```python
from build123d import *

# Parameters (mm, degrees)
SKETCH3_W           = 38.1
SKETCH3_H           = 38.1
BOSS_EXTRUDE2_DEPTH = 3.81
FILLET1_R           = 3.175
CUT_EXTRUDE1_REACH  = 65.074
SKETCH4_R           = 1.627
FILLET2_R           = 1.27
CUT_EXTRUDE2_REACH  = 64.728
SKETCH5_R           = 1.905
SKETCH7_W           = 6.35
SKETCH7_H           = 6.35
CUT_EXTRUDE4_DEPTH  = 5.08


with BuildPart() as part:
    # Sketch3 → Boss-Extrude2 (new, symmetric)
    with BuildSketch(Plane.XY):
        Polygon((34.29, -3.175), (34.29, 3.175), (26.67, 3.175), (26.67, 41.275), (34.29, 41.275), (34.29, 47.625), (13.97, 47.625), (13.97, 52.3875), (4.445, 52.3875), (4.445, 47.625), (-4.445, 47.625), (-4.445, 52.3875), (-13.97, 52.3875), (-13.97, 47.625), (-34.29, 47.625), (-34.29, 41.275), (-26.67, 41.275), (-26.67, 3.175), (-34.29, 3.175), (-34.29, -3.175), (-19.05, -3.175), (-19.05, 0), (19.05, 0), (19.05, -3.175), align=None)
        with Locations((0, 22.225)):
            Rectangle(SKETCH3_W, SKETCH3_H, mode=Mode.SUBTRACT)
    extrude(amount=BOSS_EXTRUDE2_DEPTH, both=True)

    # Fillet1
    fillet1_edges = [part.edges().sort_by_distance(p)[0] for p in [
        (34.29, 3.175, 0),
        (34.29, 41.275, 0),
        (34.29, 47.625, 0),
        (-34.29, 3.175, 0),
        (-34.29, 41.275, 0),
        (34.29, -3.175, 0),
        (-34.29, -3.175, 0),
        (-34.29, 47.625, 0),
    ]]
    fillet(fillet1_edges, radius=FILLET1_R - 0.0001)  # a hair under: the kernel refuses the full size

    # Sketch4 → Cut-Extrude1 (cut, up to next)
    with BuildSketch(Plane.XY.offset(3.81), mode=Mode.PRIVATE) as cut_extrude1_sk1:
        with Locations((-31.115, 44.45)):
            Circle(SKETCH4_R)
    cut_extrude1_tool1 = extrude(cut_extrude1_sk1.sketch, amount=-CUT_EXTRUDE1_REACH, mode=Mode.PRIVATE) & part.part
    # Sketch4 → Cut-Extrude1 (cut, up to next)
    with BuildSketch(Plane.XY.offset(3.81), mode=Mode.PRIVATE) as cut_extrude1_sk2:
        with Locations((-31.115, 0)):
            Circle(SKETCH4_R)
    cut_extrude1_tool2 = extrude(cut_extrude1_sk2.sketch, amount=-CUT_EXTRUDE1_REACH, mode=Mode.PRIVATE) & part.part
    cut_extrude1_1 = cut_extrude1_tool1.solids().sort_by_distance((-31.115, 44.45, 3.81))[0]
    add(cut_extrude1_1, mode=Mode.SUBTRACT)
    cut_extrude1_2 = cut_extrude1_tool2.solids().sort_by_distance((-31.115, 0, 3.81))[0]
    add(cut_extrude1_2, mode=Mode.SUBTRACT)
    cut_extrude1 = cut_extrude1_1 + cut_extrude1_2  # Cut-Extrude1 as one shape, for the pattern or mirror that repeats it

    # Mirror1: Cut-Extrude1 across plane
    add(cut_extrude1.mirror(Plane(origin=(0, 0, 0), x_dir=(0, 0, 1), z_dir=(1, 0, 0))), mode=Mode.SUBTRACT)

    # Fillet2
    fillet2_edges = [part.edges().sort_by_distance(p)[0] for p in [
        (-26.67, 22.225, -3.81),
        (26.67, 22.225, -3.81),
        (-13.97, 47.625, 0),
        (-13.97, 52.3875, 0),
        (-4.445, 52.3875, 0),
        (-4.445, 47.625, 0),
        (4.445, 52.3875, 0),
        (13.97, 52.3875, 0),
        (26.67, 22.225, 3.81),
        (13.97, 47.625, 0),
        (-19.05, 22.225, -3.81),
        (0, 3.175, -3.81),
        (-19.05, 3.175, 0),
        (19.05, 22.225, -3.81),
        (19.05, 3.175, 0),
        (-19.05, 22.225, 3.81),
        (0, 3.175, 3.81),
        (19.05, 22.225, 3.81),
        (-26.67, 22.225, 3.81),
    ]]
    fillet(fillet2_edges, radius=FILLET2_R)

    # Sketch5 → Cut-Extrude2 (cut, up to next)
    with BuildSketch(Plane.XZ, mode=Mode.PRIVATE) as cut_extrude2_sk1:
        with Locations((-15.24, 0)):
            Circle(SKETCH5_R)
    cut_extrude2_tool1 = extrude(cut_extrude2_sk1.sketch, amount=-CUT_EXTRUDE2_REACH, mode=Mode.PRIVATE) & part.part
    # Sketch5 → Cut-Extrude2 (cut, up to next)
    with BuildSketch(Plane.XZ, mode=Mode.PRIVATE) as cut_extrude2_sk2:
        with Locations(Location((15.24, 0, 0), (0, 0, 180))):
            Circle(SKETCH5_R)
    cut_extrude2_tool2 = extrude(cut_extrude2_sk2.sketch, amount=-CUT_EXTRUDE2_REACH, mode=Mode.PRIVATE) & part.part
    add(cut_extrude2_tool1.solids().sort_by_distance((-15.24, 0, 0))[0], mode=Mode.SUBTRACT)
    add(cut_extrude2_tool2.solids().sort_by_distance((15.24, 0, 0))[0], mode=Mode.SUBTRACT)

    # Sketch7 → Cut-Extrude4 (cut)
    with BuildSketch(Plane.XY.offset(3.81)):
        with Locations((-9.2075, 47.625)):
            Rectangle(SKETCH7_W, SKETCH7_H)
    cut_extrude4 = extrude(amount=-CUT_EXTRUDE4_DEPTH, mode=Mode.SUBTRACT)

    # Mirror2: Cut-Extrude4 across plane
    add(cut_extrude4.mirror(Plane(origin=(0, 0, 0), x_dir=(0, 0, 1), z_dir=(1, 0, 0))), mode=Mode.SUBTRACT)


solid = part.part
```
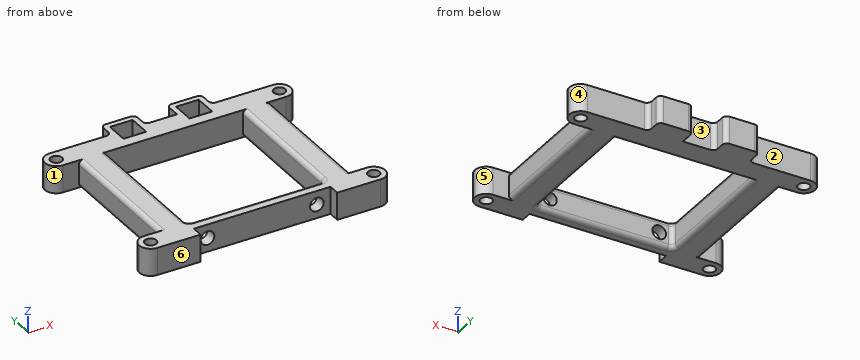
Check sheet for the modelled part. Datum: model origin and axes. Units: mm. Face numbers are marked on the shaded views. A direction names the side the tool comes from. Coordinates: 2 decimals unless noted, no trailing zeros. Write each loop counter-clockwise with the first axis right and the second up, starting at its lowest first coordinate (ties: lowest second). Pieces come first, ordered by that corner, then holes. Notation, with made-up numbers: (68.5, -21.75) -> (81.5, -21.75) arc R10 cw to (81.5, -10.75) -> close; hole circle Ø11 at (76, 16.5). An arc over 180 degrees is marked (long way). Use a Markdown table: item, result.
1. Sectioned sample at A-A (y = 22). Enter the section's corners in (x, z).
Reported:
| item | result |
|---|---|
| outline | (-26.67, -2.54) arc R1.27 ccw to (-25.4, -3.81) -> (-20.32, -3.81) arc R1.27 ccw to (-19.05, -2.54) -> (-19.05, 2.54) arc R1.27 ccw to (-20.32, 3.81) -> (-25.4, 3.81) arc R1.27 ccw to (-26.67, 2.54) -> close; (19.05, -2.54) arc R1.27 ccw to (20.32, -3.81) -> (25.4, -3.81) arc R1.27 ccw to (26.67, -2.54) -> (26.67, 2.54) arc R1.27 ccw to (25.4, 3.81) -> (20.32, 3.81) arc R1.27 ccw to (19.05, 2.54) -> close |
2. Release check for a two-part mould opening along Y. For the marked faces 4, 5 and 6 record: pulls with the +Y half, pulls with the -Y half, needs draft (parallel to the pull), parting line crosses it, or undercut.
Reported:
| item | result |
|---|---|
| face 4 | pulls with the +Y half |
| face 5 | undercut |
| face 6 | pulls with the -Y half |
3. Scan lines: line 1 along Y through (x, z) = (-31, -3) (3 decimals); line 2 along Y through (x, z) = (-16, -2.75) (3 decimals); line 3 along Z through (x, y) = (15.24, 1.6) (3 decimals). Record each from-to range of solid material in increasing order.
Reported:
| item | result |
|---|---|
| line 1 | y = -3.175 to -1.623, 1.623 to 3.175, 41.275 to 42.827, 46.073 to 47.625 |
| line 2 | y = 0 to 3.158, 41.275 to 47.625 |
| line 3 | z = -3.81 to -1.905, 1.905 to 3.81 |
4. Tool access check on the marked faces 1, 2 and 3. Record the directions out of +Z, -Z, +X, -X, +Y, -Y that give a thin tool (end or side, any length) a straight path to the whole face; none if there is none.
Reported:
| item | result |
|---|---|
| face 1 | +Z, -Z, -X |
| face 2 | +Z, -Z, -X, +Y |
| face 3 | +Z, -Z, +Y |
5. Go/stop test with flat-tipped pins: pin 1 Ø1.5 at (y, z) = (47.5, 2.5) entering from +X; pin 2 Ø2.5 at (x, z) = (10, 1) entering from -Y; pin 3 Ø1.5 at (y, z) = (16, -0.5) entering from -X. Record where each tip stops, or that it passes through.
Reported:
| item | result |
|---|---|
| pin 1 | stops at x = 33.3 |
| pin 2 | stops at y = 0 |
| pin 3 | stops at x = -26.67 |
6. Sectioned sample at C-C (z = 0). Give the number of separate pieces and of enclosed holes in the cut face, plus the area to 3 significant figures.
Reported:
| item | result |
|---|---|
| separate pieces | 2 |
| enclosed holes | 6 |
| area | 1,270 mm2 |
